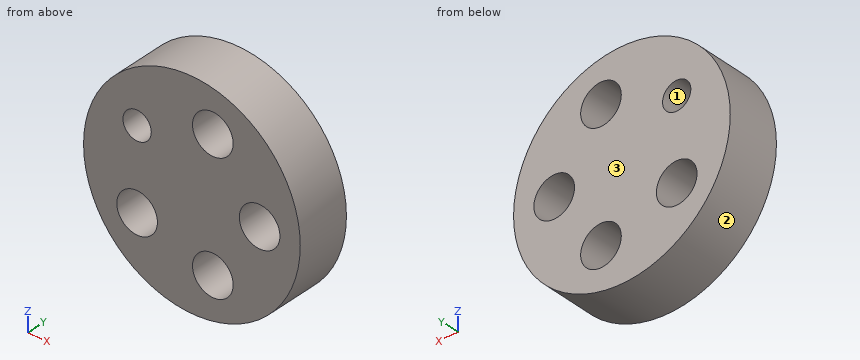
from build123d import *

# Parameters (mm, degrees)
F0_R      = 50.8
F1_DEPTH  = 25.4
F3_D      = 19.05
F4_R      = 6.634992
F5_DEPTH  = 25.4
F6_R      = 3.175
F7_DEPTH  = 25.4
F5_FACE_R = 6.634992
F8_DEPTH  = 101.6


with BuildPart() as f1:
    # F0 (on Front) → F1 (new body)
    with BuildSketch(Plane.XZ):
        Circle(F0_R)
        Polygon((15.875, 27.496307), (31.75, 0), (15.875, -27.496307), (-15.875, -27.496307), (-31.75, 0), (-15.875, 27.496307), align=None, mode=Mode.SUBTRACT)
        Polygon((15.875, -27.496307), (31.75, 0), (15.875, 27.496307), (-15.875, 27.496307), (-31.75, 0), (-15.875, -27.496307), align=None)
    extrude(amount=F1_DEPTH)

    # F3 (through all)
    with Locations(Plane.XZ.offset(25.4)):
        with Locations((9.81129, 30.196044), (31.75, 0), (-25.68629, -18.662182), (9.81129, -30.196044)):
            Hole(F3_D / 2)

    # F4 (on face) → F5 (join)
    with BuildSketch(Plane.XZ.offset(25.4)):
        with Locations((-25.68629, 18.662182)):
            Circle(F4_R)
    extrude(amount=F5_DEPTH)

    # F6 (on face) → F7 (join)
    with BuildSketch(Plane.XZ.offset(25.4)):
        with Locations((-25.68629, 18.662182)):
            Circle(F6_R)
    extrude(amount=F7_DEPTH)

    # F5_face (on face) → F8 (cut)
    with BuildSketch(Plane(origin=(-25.68629, -50.8, 18.662182), x_dir=(1, 0, 0), z_dir=(0, -1, 0))):
        Circle(F5_FACE_R)
    extrude(amount=-F8_DEPTH, mode=Mode.SUBTRACT)


solid = f1.part
CAD build for the part. Positions are in the model's coordinates, mm. Face numbers are marked on the shaded views. Coordinates: 2 decimals unless noted, no trailing zeros. Write each loop counter-clockwise with the first axis right and the second up, starting at its lowest first coordinate (ties: lowest second). Pieces come first, ordered by that corner, then holes. Notation, with made-up numbers: (-8.5, -9.75) - (48.5, -9.75) arc R24 ccw to (48.5, 2.25) - close; hole circle Ø4 at (-29, -10.5). An arc over 180 degrees is marked (long way). Use a Markdown table: item, result. Add a question column.
Item 1: Flat gauge pins, fed straight in: pin 1 (4 mm diameter, centred on x = -18.5, y = -4.5, fed in from +Z); pin 2 (1.5 mm diameter, centred on x = 37, z = -38.5, fed in from -Y); pin 3 (10 mm diameter, centred on x = 9.5, y = -16.5, fed in from +Z); pin 4 (5 mm diameter, centred on x = 14.5, y = -18.5, fed in from +Z). Where does each tip first touch, or does it go through?
Item 2: Band-saw the part on A-A, the plane z = 0. Give the cut face in (x, y) (3 decimals).
Item 3: Band-saw the part on C-C, the plane x = 31.75. Give the cut face in (y, z) (3 decimals), and give its area (3 significant figures).
Item 4: Mould opens along Z. For the marked faces 1, 2 and 3 say: pulls with the +Z half, pulls with the -Z half, needs draft (parallel to the pull), parting line crosses it, or undercut.
Item 5: Band-saw the part on B-B, the plane x = 17.5. Give the cut face in (y, z), and give its area (3 significant figures).
Item 6: Drill centre lines: L1, parallel to Z at x = 18.5, y = -11.25; L2, parallel to Z at x = -24.5, y = -8; L3, parallel to X at y = -10.75, z = 23.5. Where is each one in solid material? Low to high. Write a range as from..to.
Item 7: Band-saw the part on D-D, the plane y = -21.5. Give the cut face in (x, z) (3 decimals).
Numbers:
| question | item | result |
|---|---|---|
| 1 | pin 1 | z = 48.05 |
| 1 | pin 2 | through |
| 1 | pin 3 | z = 50.6 |
| 1 | pin 4 | z = 49.36 |
| 2 | outline | (-50.8, -25.4) - (22.225, -25.4) - (22.225, 0) - (-50.8, 0) - close; (41.275, -25.4) - (50.8, -25.4) - (50.8, 0) - (41.275, 0) - close |
| 3 | outline | (-25.4, -39.656) - (0, -39.656) - (0, -9.525) - (-25.4, -9.525) - close; (-25.4, 9.525) - (0, 9.525) - (0, 39.656) - (-25.4, 39.656) - close |
| 3 | area | 1,530 mm2 |
| 4 | face 1 | undercut |
| 4 | face 2 | parting line crosses it |
| 4 | face 3 | needs draft |
| 5 | outline | (-25.4, -47.69) - (0, -47.69) - (0, -35.82) - (-25.4, -35.82) - close; (-25.4, -24.57) - (0, -24.57) - (0, 24.57) - (-25.4, 24.57) - close; (-25.4, 35.82) - (0, 35.82) - (0, 47.69) - (-25.4, 47.69) - close |
| 5 | area | 1,850 mm2 |
| 6 | L1 | -47.31..-34.1, -26.29..26.29, 34.1..47.31 |
| 6 | L2 | -44.5..-28.11, -9.21..12.13, 25.19..44.5 |
| 6 | L3 | -45.04..-30.23, -21.15..3.04, 16.59..45.04 |
| 7 | outline | circle Ø101.6 at (0, 0); hole circle Ø19.05 at (-25.686, -18.662); hole circle Ø13.27 at (-25.686, 18.662); hole circle Ø19.05 at (9.811, -30.196); hole circle Ø19.05 at (9.811, 30.196); hole circle Ø19.05 at (31.75, 0) |
